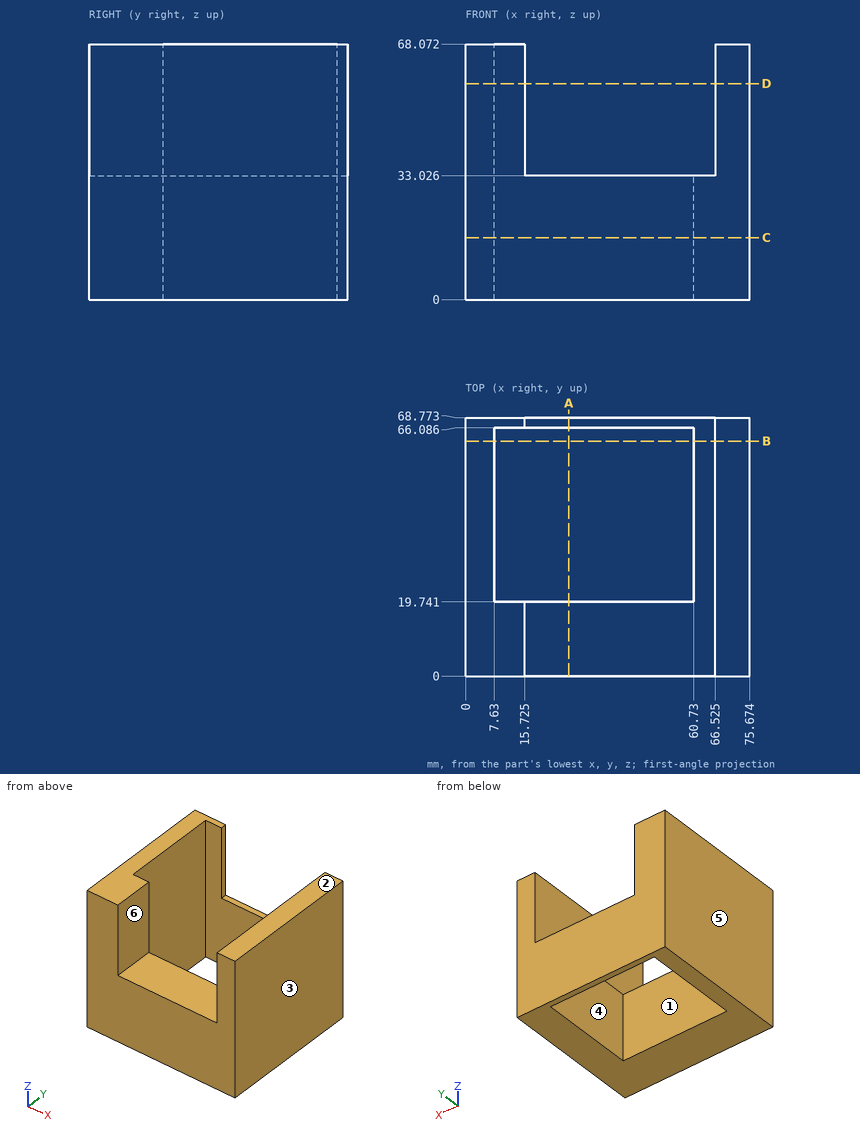
Study the drawing (mm; zero at the part's minimum x, y, z) and answer. A direction names the side the tool comes from. Give positions to 0.01 mm unless a question says otherwise; leave off trailing zeros. Write each loop counter-clockwise with the first axis right and the second up, starting at its lowest first coordinate (ties: lowest second). Pieces come first, ordered by that corner, then holes. Notation, with made-up numbers: (-28, 22.5) - (3, 22.5) arc R10 cw to (3, 27.5) - close; hole circle Ø3 at (47.5, -38). An arc over 180 degrees is marked (long way). Write item = value, one per line. Start each with the question number.
Item 1: A tool of negligible diameter and unlimited length cuts with its end or side. For the marked faces 4, 5 and 6, from which of +Z, -Z, +X, -X, +Y, -Y can it reach the whole face along a straight path? Write none if from no direction.
Item 2: Find section D-D (z = 57.5). Give the vertices of the cut face in (x, y) (1 decimal).
Item 3: Find section A-A (x = 27.5). Give the vertices of the cut face in (y, z) (1 decimal).
Item 4: Find the intervals of material crossed by probe 1 along Y at (x, z) = (53.5, 24.5) (1 decimal); probe 2 along X at (y, z) = (7, 44) (1 decimal); probe 3 along X at (y, z) = (60, 39.5) (1 decimal), in increasing order. Write a range as [from, to].
Item 5: Find section B-B (y = 62.5). Give the vertices of the cut face in (x, z) (1 decimal), then the cut area to 3 significant figures.
Item 6: The mould has two halves that part along X. Classify the marked faces 1, 2 and 3: +X half, -X half, draft (parallel to the pull), parting line (faces both ways), or undercut.
Item 7: This flat-tipped pin is pushed along its axis until it touches: P1, Ø10, axis at y = 41, z = 19, coming from the -X side. Where does it stop, or does it pass through?
Item 8: Find section C-C (z = 16.5). Give the vertices of the cut face in (x, y) (1 decimal), then the cut area to 3 significant figures.
Response:
q1.face_4 = +Z, -Z
q1.face_5 = +Z, -Z, -X, +Y, -Y
q1.face_6 = +Z, +Y, -Y
q2.outline = (0, 0) - (15.7, 0) - (15.7, 19.7) - (7.6, 19.7) - (7.6, 66.1) - (15.7, 66.1) - (15.7, 68.8) - (0, 68.8) - close; (66.5, 0) - (75.7, 0) - (75.7, 68.8) - (66.5, 68.8) - close
q3.outline = (0, 0) - (19.7, 0) - (19.7, 33) - (0, 33) - close; (66.1, 0) - (68.8, 0) - (68.8, 33) - (66.1, 33) - close
q4.probe_1 = [0, 19.7], [66.1, 68.8]
q4.probe_2 = [0, 15.7], [66.5, 75.7]
q4.probe_3 = [0, 7.6], [66.5, 75.7]
q5.outline = (0, 0) - (7.6, 0) - (7.6, 68.1) - (0, 68.1) - close; (60.7, 0) - (75.7, 0) - (75.7, 68.1) - (66.5, 68.1) - (66.5, 33) - (60.7, 33) - close
q5.area = 1,330 mm²
q6.face_1 = undercut
q6.face_2 = draft
q6.face_3 = +X half
q7.P1 = 0
q8.outline = (0, 0) - (75.7, 0) - (75.7, 68.8) - (0, 68.8) - close; hole (7.6, 19.7) - (60.7, 19.7) - (60.7, 66.1) - (7.6, 66.1) - close
q8.area = 2,740 mm²
